Autodesk Inventor part; units mm, degrees
ref_plane "YZ Plane" through (0, 0, 0) normal (1, 0, 0) x (0, 1, 0)
ref_plane "XZ Plane" through (0, 0, 0) normal (0, 1, 0) x (-1, 0, 0)
ref_plane "XY Plane" through (0, 0, 0) normal (0, 0, 1) x (1, 0, 0)
sketch "Sketch1" plane through (0, 0, 0) normal (0, 1, 0) x (-1, 0, 0)
  line L0 (0, 0) -> (78, 0)
  line L1 (78, 0) -> (78, 20)
  line L2 (78, 20) -> (0, 20)
  line L3 (0, 20) -> (0, 0)
  line L4 (39, 10) -> (68, 10)
  line L5 (39, 10) -> (10, 10)
  circle A0 centre (10, 10) radius 4
  circle A1 centre (68, 10) radius 4
  dimension "d0" = 78
  dimension "d1" = 20
  dimension "d2" = 29
  dimension "d3" = 29
  dimension "d4" = 8
  dimension "d5" = 8
extrude "Extrusion1" add sketch "Sketch1" along normal blind 10
sketch "Sketch2" plane through (-78, 0, 20) normal (0, 0, 1) x (1, 0, 0)
  line L0 (0, 10) -> (78, 10)
  circle A0 centre (39, 10) radius 4
  dimension "d8" = 8
extrude "Extrusion2" cut sketch "Sketch2" against normal blind 20
properties part number "Z_MotorMount_RodHolder_Part2_V2" material "Birch"
Check sheet for the modelled part. Datum: model origin and axes. Units: mm. Round coordinates to 2 decimals unless told otherwise and drop trailing zeros. Loops run counter-clockwise (first coordinate to the right, second up) from the corner with the lowest first, then second, coordinate; pieces in that order, holes last.
1. Mould release check, pull along X, two halves, no side actions. Record for faces 1 (the flat face through (-60, 10, 10)), 2 (the flat face through (0, 5, 10)), 3 (the cylindrical face through (-6.8, 4.9, 12.4)), 4 (the flat face through (-78, 5, 10)): released by +X, released by -X, zero draft, split by the parting line, or undercut.
2. Sectioned sample at B-B on z = 10. Record the boundary of the cut face in (x, y).
3. Sectioned sample at C-C on y = 7.25. Record the boundary of the cut face in (x, z), and give its area (3 significant figures).
4. Sectioned sample at D-D on y = 2.75. Record the boundary of the cut face in (x, z).
5. Sectioned sample at A-A on x = -10. Record the boundary of the cut face in (y, z), and give its area (3 significant figures).
6. Scan lines: probe 1 along Z at (x, y) = (-68, 6); probe 2 along X at (y, z) = (4, 11); probe 3 along X at (y, z) = (5.5, 12). Record each from-to range of solid material in increasing order.
Recorded:
1. face 1: zero draft
1. face 2: released by +X
1. face 3: undercut
1. face 4: released by -X
2. outline: (-78, 0) - (-72, 0) - (-72, 10) - (-78, 10) - close; (-64, 0) - (-14, 0) - (-14, 10) - (-35, 10) arc R4 cw to (-43, 10) - (-64, 10) - close; (-6, 0) - (0, 0) - (0, 10) - (-6, 10) - close
3. outline: (-78, 0) - (-41.9, 0) - (-41.9, 20) - (-78, 20) - close; (-36.1, 0) - (0, 0) - (0, 20) - (-36.1, 20) - close; hole circle Ø8 at (-68, 10); hole circle Ø8 at (-10, 10)
3. area: 1,340 mm2
4. outline: (-78, 0) - (0, 0) - (0, 20) - (-78, 20) - close; hole circle Ø8 at (-68, 10); hole circle Ø8 at (-10, 10)
5. outline: (0, 0) - (10, 0) - (10, 6) - (0, 6) - close; (0, 14) - (10, 14) - (10, 20) - (0, 20) - close
5. area: 120 mm2
6. probe 1: z = 0 to 6, 14 to 20
6. probe 2: x = -78 to -71.87, -64.13 to -13.87, -6.13 to 0
6. probe 3: x = -78 to -71.46, -64.54 to -13.46, -6.54 to 0
